Could you check a few things on this drawing? It's one solid part, dimensions in mm from its lowest x, y, z. A direction names the side the tool comes from. Coordinates: 2 decimals unless noted, no trailing zeros. Loops run counter-clockwise (first coordinate to the right, second up) from the corner with the lowest first, then second, coordinate; pieces in that order, holes last.
1) Imagine slicing it at C-C on z = 6.25. Give the number of separate pieces and of enclosed holes in the cut face, plus the area to 3 significant figures.
2) For the marked faces 1, 2 and 3, which set-ups out of +Z, -Z, +X, -X, +Y, -Y let a thin tool reach every point of the face, with its end or its side?
3) Imagine slicing it at B-B on y = 34. Please give me the cut outline in (x, z) (3 decimals).
4) Will these pins go through, and if not, where does the flat tip stop? P1, Ø4, axis at x = 4, z = 10, coming from the +Y side (3 decimals); P2, Ø3, axis at y = 6.5, z = 8.5, coming from the +X side; P3, Ø2.5, axis at x = 2.5, z = 5, coming from the -Y side (3 decimals).
5) If I drill on line 1 along Y through (x, z) = (19, 3.5) (3 decimals); line 2 along X through (y, z) = (7, 11) (3 decimals), over which ranges is the centre line in solid material (lowest first)?
6) Imagine slicing it at A-A on x = 49. Please give me the cut outline in (y, z) (3 decimals).
7) Thinking about a two-plate mould opening in Y: for the marked faces 4, 5, 6 and 7, which applies, released by +Y, released by -Y, zero draft, split by the parting line, or undercut?
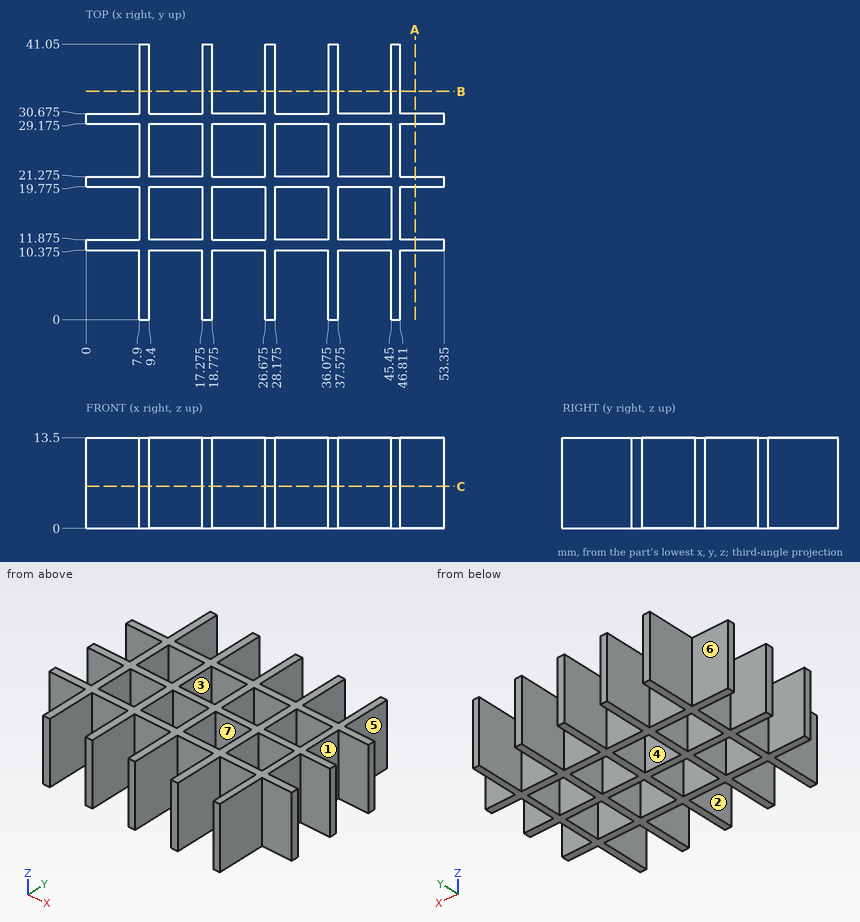
Filled in:
1. separate pieces: 1
1. enclosed holes: 8
1. area: 509 mm2
2. face 1: +Z, -Z, +X
2. face 2: +Z, -Z, -Y
2. face 3: +Z, -Z
3. outline: (7.9, 0) - (9.4, 0) - (9.4, 13.5) - (7.9, 13.5) - close; (17.275, 0) - (18.775, 0) - (18.775, 13.5) - (17.275, 13.5) - close; (26.675, 0) - (28.175, 0) - (28.175, 13.5) - (26.675, 13.5) - close; (36.075, 0) - (37.575, 0) - (37.575, 13.5) - (36.075, 13.5) - close; (45.45, 0) - (46.811, 0) - (46.811, 13.5) - (45.45, 13.5) - close
4. P1: stops at y = 30.675
4. P2: stops at x = 46.81
4. P3: stops at y = 10.375
5. line 1: y = 10.375 to 11.875, 19.775 to 21.275, 29.175 to 30.675
5. line 2: x = 7.9 to 9.4, 17.275 to 18.775, 26.675 to 28.175, 36.075 to 37.575, 45.45 to 46.811
6. outline: (10.375, 0) - (11.875, 0) - (11.875, 13.5) - (10.375, 13.5) - close; (19.775, 0) - (21.275, 0) - (21.275, 13.5) - (19.775, 13.5) - close; (29.175, 0) - (30.675, 0) - (30.675, 13.5) - (29.175, 13.5) - close
7. face 4: undercut
7. face 5: zero draft
7. face 6: released by +Y
7. face 7: undercut
